from build123d import *

# Parameters (mm, degrees)
F0_W     = 100
F0_H     = 70
F1_DEPTH = 107
F2_R     = 37.5
F3_DEPTH = 61.2
F4_R     = 14.4000008702
F5_DEPTH = 131.201
F6_SIZE  = 5


with BuildPart() as f1:
    # F0 (on Front) → F1 (new body)
    with BuildSketch(Plane.XZ):
        with Locations((50, 35)):
            Rectangle(F0_W, F0_H)
    extrude(amount=F1_DEPTH)

    # F2 (on face) → F3 (join)
    with BuildSketch(Plane.XY.offset(70)):
        with Locations((50, -57)):
            Circle(F2_R)
    extrude(amount=F3_DEPTH)

    # F4 (on face) → F5 (cut, through all)
    with BuildSketch(Plane.XY.offset(131.2)):
        with Locations((50, -57)):
            Circle(F4_R)
    extrude(amount=-F5_DEPTH, mode=Mode.SUBTRACT)

    # F6
    f6_edges = [f1.edges().sort_by_distance(p)[0] for p in [
        (12.5, -57, 131.2),
        (35.599999, -57, 131.2),
    ]]
    chamfer(f6_edges, length=F6_SIZE)


solid = f1.part
Check sheet for the modelled part. Datum: model origin and axes. Units: mm. A direction names the side the tool comes from. Coordinates: 2 decimals unless noted, no trailing zeros. Loops run counter-clockwise (first coordinate to the right, second up) from the corner with the lowest first, then second, coordinate; pieces in that order, holes last. Notation, with made-up numbers: (-37.5, 48) -> (5.5, 48) arc R31 ccw to (5.5, 81) -> close; hole circle Ø9 at (-25, 68.25). An arc over 180 degrees is marked (long way). Write item = value, one per line. Start each with the question number.
1. Material ranges on line 1 (Y direction, x = 50, z = 92.5); line 2 (Y direction, x = 50, z = 36.5); line 3 (X direction, y = -56, z = 87), recorded low to high.
2. Tool access check on faces 1 (the flat face through (49, -17, 70)), 2 (the flat face through (49, -107, 35)). Record the directions out of +Z, -Z, +X, -X, +Y, -Y that give a thin tool (end or side, any length) a straight path to the whole face; none if there is none.
3. Draft check along Y on faces 3 (the conical face through (46.81, -71.36, 126.51)), 4 (the conical face through (81.231, -47.165, 130.957)), 5 (the flat face through (49, -41, 0)). Enter one of: released by +Y, released by -Y, zero draft, split by the parting line, or undercut.
4. Section check A-A on x = 50. Record the cut outline in (y, z), then the cut area to 3 significant figures.
5. Section check B-B on y = -57. Record the cut outline in (x, z).
6. Section check C-C on z = 29.5. Record the cut outline in (x, y), then the cut area to 3 significant figures.
7. Section check D-D on y = -10.5. Record the cut outline in (x, z).
8. Depth check by flat-ended pin: P1, Ø2, axis at y = -20.5, z = 62, coming from the -X side; P2, Ø1.5, axis at y = -67, z = 108.5, coming from the -X side; P3, Ø12, axis at y = -67.5, z = 96, coming from the -X side; P4, Ø8, axis at y = -59.5, z = 115, coming from the +X side. Enter the tip coordinate at first touch or a pass-through.
Responses:
q1.line_1 = -94.5 to -71.4, -42.6 to -19.5
q1.line_2 = -107 to -71.4, -42.6 to 0
q1.line_3 = 12.51 to 35.63, 64.37 to 87.49
q2.face_1 = +Z
q2.face_2 = +Z, -Z, +X, -X, -Y
q3.face_3 = undercut
q3.face_4 = split by the parting line
q3.face_5 = zero draft
q4.outline = (-107, 0) -> (-71.4, 0) -> (-71.4, 126.2) -> (-76.4, 131.2) -> (-89.5, 131.2) -> (-94.5, 126.2) -> (-94.5, 70) -> (-107, 70) -> close; (-42.6, 0) -> (0, 0) -> (0, 70) -> (-19.5, 70) -> (-19.5, 126.2) -> (-24.5, 131.2) -> (-37.6, 131.2) -> (-42.6, 126.2) -> close
q4.area = 8,250 mm2
q5.outline = (0, 0) -> (35.6, 0) -> (35.6, 126.2) -> (30.6, 131.2) -> (17.5, 131.2) -> (12.5, 126.2) -> (12.5, 70) -> (0, 70) -> close; (64.4, 0) -> (100, 0) -> (100, 70) -> (87.5, 70) -> (87.5, 126.2) -> (82.5, 131.2) -> (69.4, 131.2) -> (64.4, 126.2) -> close
q6.outline = (0, -107) -> (100, -107) -> (100, 0) -> (0, 0) -> close; hole circle Ø28.8 at (50, -57)
q6.area = 10,000 mm2
q7.outline = (0, 0) -> (100, 0) -> (100, 70) -> (0, 70) -> close
q8.P1 = 0
q8.P2 = 13.66
q8.P3 = 12.77
q8.P4 = 87.5
